For this review, take the finished solid that the model builds, in its own axes (mm). Face numbers are marked on the shaded views. A direction names the side the tool comes from. Coordinates: 2 decimals unless noted, no trailing zeros. Order: outer loops, then holes, each group sorted by start corner. A loop starts at its lowest first (then second) coordinate and runs counter-clockwise, first axis right, second up.
from build123d import *

# Parameters (mm, degrees)
SKETCH1_W           = 5
SKETCH1_H           = 8
BOSS_EXTRUDE3_DEPTH = 59
SKETCH8_W           = 5
SKETCH8_H           = 1
BOSS_EXTRUDE5_DEPTH = 1
SKETCH10_W          = 5
SKETCH10_H          = 1
BOSS_EXTRUDE7_DEPTH = 1
SKETCH6_W           = 5
SKETCH6_H           = 31
CUT_EXTRUDE1_DEPTH  = 2


with BuildPart() as part:
    # Sketch1 → Boss-Extrude3 (new body)
    with BuildSketch(Plane.XY):
        Rectangle(SKETCH1_W, SKETCH1_H)
        with BuildLine():
            Line((-1.5, 2), (-1.5, -2))
            ThreePointArc((-1.5, -2), (-1.207106781, -2.707106781), (-0.5, -3))
            Line((-0.5, -3), (-0.5, 3))
            ThreePointArc((-0.5, 3), (-1.207106781, 2.707106781), (-1.5, 2))
        make_face(mode=Mode.SUBTRACT)
        with BuildLine():
            Line((1.5, 2), (1.5, -2))
            ThreePointArc((1.5, -2), (1.207106781, -2.707106781), (0.5, -3))
            Line((0.5, -3), (0.5, 3))
            ThreePointArc((0.5, 3), (1.207106781, 2.707106781), (1.5, 2))
        make_face(mode=Mode.SUBTRACT)
    extrude(amount=BOSS_EXTRUDE3_DEPTH)

    # Sketch8 → Boss-Extrude5 (add)
    with BuildSketch(Plane.XZ.offset(4)):
        with Locations((0, 11.5)):
            Rectangle(SKETCH8_W, SKETCH8_H)
    extrude(amount=BOSS_EXTRUDE5_DEPTH)

    # Sketch10 → Boss-Extrude7 (add)
    with BuildSketch(Plane.XZ.offset(4)):
        with Locations((0, 46)):
            Rectangle(SKETCH10_W, SKETCH10_H)
    extrude(amount=BOSS_EXTRUDE7_DEPTH)

    # Sketch6 → Cut-Extrude1 (cut)
    with BuildSketch(Plane(origin=(0, 4, 0), x_dir=(1, 0, 0), z_dir=(0, 1, 0))):
        with Locations((0, -15.5)):
            Rectangle(SKETCH6_W, SKETCH6_H)
    extrude(amount=-CUT_EXTRUDE1_DEPTH, mode=Mode.SUBTRACT)


solid = part.part
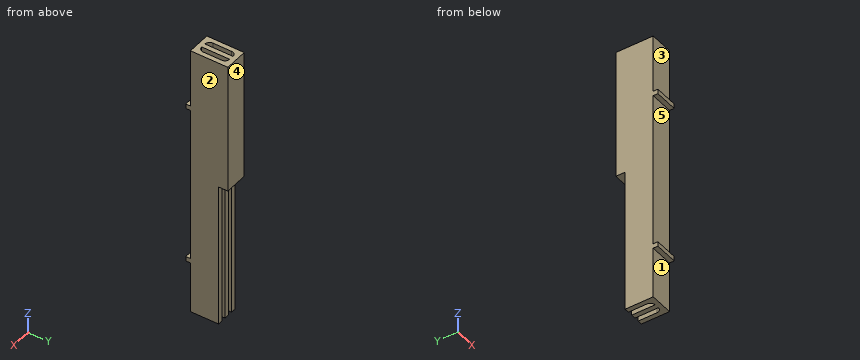
1. Machinability: for the marked faces 1, 2, 3, 4 and 5, which of the approach directions +Z, -Z, +X, -X, +Y, -Y give a long, thin tool a straight path to every point of the face, cutting with its end or side? Answer none if there is none.
Answer below:
face 1: -Z, +X, -X, -Y
face 2: +Z, -Z, +X, +Y, -Y
face 3: +Z, +X, -X, -Y
face 4: +Z, -Z, +X, -X, +Y
face 5: +X, -X, -Y
2. Take a section at C-C, the plane x = -2. Give the boundary of the cut face in (y, z).
Answer below:
outline: (-5, 11) - (-4, 11) - (-4, 0) - (2, 0) - (2, 31) - (4, 31) - (4, 59) - (-4, 59) - (-4, 46.5) - (-5, 46.5) - (-5, 45.5) - (-4, 45.5) - (-4, 12) - (-5, 12) - close
3. Clearance check with flat-ended pins moving along their axes: pin 1 Ø0.8 at (x, y) = (-1, -4.5) entering from -Z; pin 2 Ø0.8 at (x, z) = (-2, 13) entering from +Y; pin 3 Ø0.6 at (x, y) = (-1, 3) entering from -Z. State where each tip first meets the part, or that it passes through.
Answer below:
pin 1: stops at z = 11
pin 2: stops at y = 2
pin 3: stops at z = 31
4. Take a section at D-D, the plane z = 24. Give the boundary of the cut face in (x, y).
Answer below:
outline: (-2.5, -4) - (2.5, -4) - (2.5, 2) - (1.5, 2) - (1.5, -2) arc R1 cw to (0.5, -3) - (0.5, 2) - (-0.5, 2) - (-0.5, -3) arc R1 cw to (-1.5, -2) - (-1.5, 2) - (-2.5, 2) - close
5. Take a section at B-B, the plane y = 1. Give the boundary of the cut face in (x, z), plus the area to 3 significant figures.
Answer below:
outline: (-2.5, 0) - (-1.5, 0) - (-1.5, 59) - (-2.5, 59) - close; (-0.5, 0) - (0.5, 0) - (0.5, 59) - (-0.5, 59) - close; (1.5, 0) - (2.5, 0) - (2.5, 59) - (1.5, 59) - close
area: 177 mm2
6. To check wall thickness, follow L1, parallel to X at y = -2, z = 8.5; L2, parallel to Y at x = -0.65, z = 50; L3, parallel to Z at x = 0.7, y = -4.25. State the ranges of each line that lie inside material, in increasing order.
Answer below:
L1: x = -2.5 to -1.5, -0.5 to 0.5, 1.5 to 2.5
L2: y = -4 to -2.99, 2.99 to 4
L3: z = 11 to 12, 45.5 to 46.5
7. Take a section at A-A, the plane z = 33. Give the boundary of the cut face in (x, y).
Answer below:
outline: (-2.5, -4) - (2.5, -4) - (2.5, 4) - (-2.5, 4) - close; hole (-1.5, -2) arc R1 ccw to (-0.5, -3) - (-0.5, 3) arc R1 ccw to (-1.5, 2) - close; hole (0.5, -3) arc R1 ccw to (1.5, -2) - (1.5, 2) arc R1 ccw to (0.5, 3) - close
